```python
from build123d import *

# Parameters (mm, degrees)
SKETCH1_W                       = 314
SKETCH1_H                       = 134
BOSS_EXTRUDE1_DEPTH             = 160
SKETCH2_W                       = 350
SKETCH2_H                       = 150
BOSS_EXTRUDE3_DEPTH             = 10
SKETCH3_R                       = 41
BOSS_EXTRUDE5_DEPTH             = 150
F_5_0MM_DOWEL_HOLE1_D           = 5
F_5_0MM_DOWEL_HOLE1_CSINK_D     = 5.05
F_5_0MM_DOWEL_HOLE1_CSINK_ANGLE = 100
CIRPATTERN1_COUNT               = 6
SKETCH3_3_R                     = 27.5
CUT_EXTRUDE1_DEPTH              = 151
SKETCH6_R                       = 43
BOSS_EXTRUDE6_DEPTH             = 150
SKETCH6_3_R                     = 27.5
CUT_EXTRUDE2_DEPTH              = 151
F_5_0MM_DOWEL_HOLE2_D           = 5
F_5_0MM_DOWEL_HOLE2_CSINK_D     = 5.05
F_5_0MM_DOWEL_HOLE2_CSINK_ANGLE = 100
CIRPATTERN2_COUNT               = 6
MIRROR1_COPY_1_D                = 5
MIRROR1_COPY_1_CSINK_D          = 5.05
MIRROR1_COPY_1_CSINK_ANGLE      = 100
MIRROR1_COPY_2_D                = 5
MIRROR1_COPY_2_CSINK_D          = 5.05
MIRROR1_COPY_2_CSINK_ANGLE      = 100
MIRROR1_COPY_3_D                = 5
MIRROR1_COPY_3_CSINK_D          = 5.05
MIRROR1_COPY_3_CSINK_ANGLE      = 100
MIRROR1_COPY_4_D                = 5
MIRROR1_COPY_4_CSINK_D          = 5.05
MIRROR1_COPY_4_CSINK_ANGLE      = 100
MIRROR1_COPY_5_D                = 5
MIRROR1_COPY_5_CSINK_D          = 5.05
MIRROR1_COPY_5_CSINK_ANGLE      = 100
MIRROR2_COPY_1_D                = 5
MIRROR2_COPY_1_CSINK_D          = 5.05
MIRROR2_COPY_1_CSINK_ANGLE      = 100
MIRROR2_COPY_2_D                = 5
MIRROR2_COPY_2_CSINK_D          = 5.05
MIRROR2_COPY_2_CSINK_ANGLE      = 100
MIRROR2_COPY_3_D                = 5
MIRROR2_COPY_3_CSINK_D          = 5.05
MIRROR2_COPY_3_CSINK_ANGLE      = 100
MIRROR2_COPY_4_D                = 5
MIRROR2_COPY_4_CSINK_D          = 5.05
MIRROR2_COPY_4_CSINK_ANGLE      = 100
MIRROR2_COPY_5_D                = 5
MIRROR2_COPY_5_CSINK_D          = 5.05
MIRROR2_COPY_5_CSINK_ANGLE      = 100
SKETCH9_R                       = 12.5
BOSS_EXTRUDE7_DEPTH             = 6
CUT_EXTRUDE3_START              = 6
SKETCH9_3_R                     = 9
CUT_EXTRUDE3_DEPTH              = 30
CHAMFER1_SIZE                   = 2
SKETCH10_W                      = 26.35
SKETCH10_H                      = 43
BOSS_EXTRUDE8_DEPTH             = 25
CUT_EXTRUDE4_REACH              = 90.175
SKETCH12_R                      = 7.5
CUT_EXTRUDE5_DEPTH              = 50
CUT_EXTRUDE6_START              = -161
SKETCH13_R                      = 4
CUT_EXTRUDE6_DEPTH              = 205
MIRROR5_START                   = -161
MIRROR5_COPY_1_SKETCH_R         = 4
MIRROR5_COPY_1_DEPTH            = 205
MIRROR5_COPY_2_SKETCH_R         = 4
MIRROR5_COPY_2_DEPTH            = 205
SKETCH14_W                      = 364.166364604
SKETCH14_H                      = 92.820269588
CUT_EXTRUDE7_DEPTH              = 151
SKETCH15_W                      = 300
SKETCH15_H                      = 120
CUT_EXTRUDE9_DEPTH              = 150


with BuildPart() as part:
    # Sketch1 → Boss-Extrude1 (new body)
    with BuildSketch(Plane(origin=(0, 0, 0), x_dir=(1, 0, 0), z_dir=(0, 1, 0))):
        Rectangle(SKETCH1_W, SKETCH1_H)
    extrude(amount=BOSS_EXTRUDE1_DEPTH)

    # Sketch2 → Boss-Extrude3 (add)
    with BuildSketch(Plane(origin=(0, 160, 0), x_dir=(1, 0, 0), z_dir=(0, 1, 0))):
        Rectangle(SKETCH2_W, SKETCH2_H)
    extrude(amount=-BOSS_EXTRUDE3_DEPTH)

    # Sketch3 → Boss-Extrude5 (add, through all)
    with BuildSketch(Plane.XY.offset(75)):
        with Locations((95, 160)):
            Circle(SKETCH3_R)
    extrude(amount=-BOSS_EXTRUDE5_DEPTH)

    # Ø5.0mm Dowel Hole1 (through all)
    with Locations(Plane.XY.offset(75)):
        with Locations((95, 195)):
            f_5_0mm_dowel_hole1 = CounterSinkHole(F_5_0MM_DOWEL_HOLE1_D / 2, F_5_0MM_DOWEL_HOLE1_CSINK_D / 2, counter_sink_angle=F_5_0MM_DOWEL_HOLE1_CSINK_ANGLE)

    # CirPattern1: Ø5.0mm Dowel Hole1 ×6 about axis
    cirpattern1_axis = Axis((95, 160, 0), (0, 0, 1))
    for i in range(1, CIRPATTERN1_COUNT):
        add(f_5_0mm_dowel_hole1.rotate(cirpattern1_axis, i * 360 / CIRPATTERN1_COUNT), mode=Mode.SUBTRACT)

    # Sketch3<3> → Cut-Extrude1 (cut, through all)
    with BuildSketch(Plane.XY.offset(75)):
        with Locations((95, 160)):
            Circle(SKETCH3_3_R)
    extrude(amount=-CUT_EXTRUDE1_DEPTH, mode=Mode.SUBTRACT)

    # Sketch6 → Boss-Extrude6 (add, through all)
    with BuildSketch(Plane.XY.offset(75)):
        with Locations((-25, 160)):
            Circle(SKETCH6_R)
    extrude(amount=-BOSS_EXTRUDE6_DEPTH)

    # Sketch6<3> → Cut-Extrude2 (cut, through all)
    with BuildSketch(Plane.XY.offset(75)):
        with Locations((-25, 160)):
            Circle(SKETCH6_3_R)
    extrude(amount=-CUT_EXTRUDE2_DEPTH, mode=Mode.SUBTRACT)

    # Ø5.0mm Dowel Hole2 (through all)
    with Locations(Plane.XY.offset(75)):
        with Locations((-25, 193)):
            f_5_0mm_dowel_hole2 = CounterSinkHole(F_5_0MM_DOWEL_HOLE2_D / 2, F_5_0MM_DOWEL_HOLE2_CSINK_D / 2, counter_sink_angle=F_5_0MM_DOWEL_HOLE2_CSINK_ANGLE)

    # CirPattern2: Ø5.0mm Dowel Hole2 ×6 about axis
    cirpattern2_axis = Axis((-25, 160, 0), (0, 0, 1))
    for i in range(1, CIRPATTERN2_COUNT):
        add(f_5_0mm_dowel_hole2.rotate(cirpattern2_axis, i * 360 / CIRPATTERN2_COUNT), mode=Mode.SUBTRACT)

    # Mirror1: Ø5.0mm Dowel Hole2 across plane
    add(f_5_0mm_dowel_hole2.mirror(Plane.XY), mode=Mode.SUBTRACT)

    # Mirror1 copy 1 (through all)
    with Locations(Plane(origin=(126.064064606, 101.650635095, -75), x_dir=(0.5, 0.866025404, 0), z_dir=(0, 0, -1))):
        with Locations((-25, -193)):
            CounterSinkHole(MIRROR1_COPY_1_D / 2, MIRROR1_COPY_1_CSINK_D / 2, counter_sink_angle=MIRROR1_COPY_1_CSINK_ANGLE)

    # Mirror1 copy 2 (through all)
    with Locations(Plane(origin=(101.064064606, 261.650635095, -75), x_dir=(-0.5, 0.866025404, 0), z_dir=(0, 0, -1))):
        with Locations((-25, -193)):
            CounterSinkHole(MIRROR1_COPY_2_D / 2, MIRROR1_COPY_2_CSINK_D / 2, counter_sink_angle=MIRROR1_COPY_2_CSINK_ANGLE)

    # Mirror1 copy 3 (through all)
    with Locations(Plane(origin=(-50, 320, -75), x_dir=(-1, 0, 0), z_dir=(0, 0, -1))):
        with Locations((-25, -193)):
            CounterSinkHole(MIRROR1_COPY_3_D / 2, MIRROR1_COPY_3_CSINK_D / 2, counter_sink_angle=MIRROR1_COPY_3_CSINK_ANGLE)

    # Mirror1 copy 4 (through all)
    with Locations(Plane(origin=(-176.064064606, 218.349364905, -75), x_dir=(-0.5, -0.866025404, 0), z_dir=(0, 0, -1))):
        with Locations((-25, -193)):
            CounterSinkHole(MIRROR1_COPY_4_D / 2, MIRROR1_COPY_4_CSINK_D / 2, counter_sink_angle=MIRROR1_COPY_4_CSINK_ANGLE)

    # Mirror1 copy 5 (through all)
    with Locations(Plane(origin=(-151.064064606, 58.349364905, -75), x_dir=(0.5, -0.866025404, 0), z_dir=(0, 0, -1))):
        with Locations((-25, -193)):
            CounterSinkHole(MIRROR1_COPY_5_D / 2, MIRROR1_COPY_5_CSINK_D / 2, counter_sink_angle=MIRROR1_COPY_5_CSINK_ANGLE)

    # Mirror2: Ø5.0mm Dowel Hole1 across plane
    add(f_5_0mm_dowel_hole1.mirror(Plane.XY), mode=Mode.SUBTRACT)

    # Mirror2 copy 1 (through all)
    with Locations(Plane(origin=(186.064064606, -2.27241336, -75), x_dir=(0.5, 0.866025404, 0), z_dir=(0, 0, -1))):
        with Locations((95, -195)):
            CounterSinkHole(MIRROR2_COPY_1_D / 2, MIRROR2_COPY_1_CSINK_D / 2, counter_sink_angle=MIRROR2_COPY_1_CSINK_ANGLE)

    # Mirror2 copy 2 (through all)
    with Locations(Plane(origin=(281.064064606, 157.72758664, -75), x_dir=(-0.5, 0.866025404, 0), z_dir=(0, 0, -1))):
        with Locations((95, -195)):
            CounterSinkHole(MIRROR2_COPY_2_D / 2, MIRROR2_COPY_2_CSINK_D / 2, counter_sink_angle=MIRROR2_COPY_2_CSINK_ANGLE)

    # Mirror2 copy 3 (through all)
    with Locations(Plane(origin=(190, 320, -75), x_dir=(-1, 0, 0), z_dir=(0, 0, -1))):
        with Locations((95, -195)):
            CounterSinkHole(MIRROR2_COPY_3_D / 2, MIRROR2_COPY_3_CSINK_D / 2, counter_sink_angle=MIRROR2_COPY_3_CSINK_ANGLE)

    # Mirror2 copy 4 (through all)
    with Locations(Plane(origin=(3.935935394, 322.27241336, -75), x_dir=(-0.5, -0.866025404, 0), z_dir=(0, 0, -1))):
        with Locations((95, -195)):
            CounterSinkHole(MIRROR2_COPY_4_D / 2, MIRROR2_COPY_4_CSINK_D / 2, counter_sink_angle=MIRROR2_COPY_4_CSINK_ANGLE)

    # Mirror2 copy 5 (through all)
    with Locations(Plane(origin=(-91.064064606, 162.27241336, -75), x_dir=(0.5, -0.866025404, 0), z_dir=(0, 0, -1))):
        with Locations((95, -195)):
            CounterSinkHole(MIRROR2_COPY_5_D / 2, MIRROR2_COPY_5_CSINK_D / 2, counter_sink_angle=MIRROR2_COPY_5_CSINK_ANGLE)

    # Sketch9 → Boss-Extrude7 (add)
    with BuildSketch(Plane(origin=(157, 0, 0), x_dir=(0, 0, -1), z_dir=(1, 0, 0))):
        with Locations((0, 22.5)):
            Circle(SKETCH9_R)
    extrude(amount=BOSS_EXTRUDE7_DEPTH)

    # Sketch9<3> → Cut-Extrude3 (cut)
    with BuildSketch(Plane(origin=(157, 0, 0), x_dir=(0, 0, -1), z_dir=(1, 0, 0)).offset(CUT_EXTRUDE3_START)):
        with Locations((0, 22.5)):
            Circle(SKETCH9_3_R)
    extrude(amount=-CUT_EXTRUDE3_DEPTH, mode=Mode.SUBTRACT)

    # Chamfer1
    chamfer1_edges = [part.edges().sort_by_distance(p)[0] for p in [
        (163, 22.5, 12.5),
    ]]
    chamfer(chamfer1_edges, length=CHAMFER1_SIZE)

    # Sketch10 → Boss-Extrude8 (add)
    with BuildSketch(Plane(origin=(157, 0, 0), x_dir=(0, 0, -1), z_dir=(1, 0, 0))):
        with Locations((0, 66.5)):
            Rectangle(SKETCH10_W, SKETCH10_H)
    extrude(amount=BOSS_EXTRUDE8_DEPTH)

    # Sketch11 → Cut-Extrude4 (cut, up to next)
    with BuildSketch(Plane(origin=(0, 0, -13.175), x_dir=(-1, 0, 0), z_dir=(0, 0, -1)), mode=Mode.PRIVATE) as cut_extrude4_sk1:
        Polygon((-162, 88), (-182, 68), (-200.649139224, 72.819299993), (-183.741650688, 106.337654458), align=None)
    cut_extrude4_tool1 = extrude(cut_extrude4_sk1.sketch, amount=-CUT_EXTRUDE4_REACH, mode=Mode.PRIVATE) & part.part
    add(cut_extrude4_tool1.solids().sort_by_distance((181.949584, 85.075168, -13.175))[0], mode=Mode.SUBTRACT)

    # Sketch12 → Cut-Extrude5 (cut)
    with BuildSketch(Plane(origin=(125, 125, 0), x_dir=(0, 0, -1), z_dir=(0.707106781, 0.707106781, 0))):
        with Locations((0, -63.993163697)):
            Circle(SKETCH12_R)
    extrude(amount=-CUT_EXTRUDE5_DEPTH, mode=Mode.SUBTRACT)

    # Sketch13 → Cut-Extrude6 (cut)
    with BuildSketch(Plane(origin=(0, 160, 0), x_dir=(1, 0, 0), z_dir=(0, 1, 0)).offset(CUT_EXTRUDE6_START)):
        with Locations((-167, 67)):
            Circle(SKETCH13_R)
    cut_extrude6 = extrude(amount=CUT_EXTRUDE6_DEPTH, mode=Mode.SUBTRACT)

    # Mirror3: Cut-Extrude6 across plane
    add(cut_extrude6.mirror(Plane(origin=(0, 0, 0), x_dir=(0, 0, 1), z_dir=(1, 0, 0))), mode=Mode.SUBTRACT)

    # Mirror4: Cut-Extrude6 across plane
    add(cut_extrude6.mirror(Plane.XY), mode=Mode.SUBTRACT)

    # Mirror5 copy 1 sketch → Mirror5 copy 1 (cut)
    with BuildSketch(Plane(origin=(0, 160, 0), x_dir=(-1, 0, 0), z_dir=(0, 1, 0)).offset(MIRROR5_START)):
        with Locations((-167, 67)):
            Circle(MIRROR5_COPY_1_SKETCH_R)
    extrude(amount=MIRROR5_COPY_1_DEPTH, mode=Mode.SUBTRACT)

    # Mirror5 copy 2 sketch → Mirror5 copy 2 (cut)
    with BuildSketch(Plane(origin=(0, 160, 0), x_dir=(1, 0, 0), z_dir=(0, 1, 0)).offset(MIRROR5_START)):
        with Locations((-167, -67)):
            Circle(MIRROR5_COPY_2_SKETCH_R)
    extrude(amount=MIRROR5_COPY_2_DEPTH, mode=Mode.SUBTRACT)

    # Sketch14 → Cut-Extrude7 (cut, through all)
    with BuildSketch(Plane.XY.offset(75)):
        with Locations((7.083182302, 206.410134794)):
            Rectangle(SKETCH14_W, SKETCH14_H)
    extrude(amount=-CUT_EXTRUDE7_DEPTH, mode=Mode.SUBTRACT)

    # Sketch15 → Cut-Extrude9 (cut)
    with BuildSketch(Plane(origin=(0, 160, 0), x_dir=(1, 0, 0), z_dir=(0, 1, 0))):
        Rectangle(SKETCH15_W, SKETCH15_H)
    extrude(amount=-CUT_EXTRUDE9_DEPTH, mode=Mode.SUBTRACT)


solid = part.part
```
Part model, mm, in its own coordinate system. A direction names the side the tool comes from. Round coordinates to 2 decimals unless told otherwise and drop trailing zeros. Write each loop counter-clockwise with the first axis right and the second up, starting at its lowest first coordinate (ties: lowest second). Pieces come first, ordered by that corner, then holes. Notation, with made-up numbers: (-18.75, 78) -> (32.25, 78) arc R14 cw to (32.25, 89) -> close; hole circle Ø6 at (85.25, 9). An arc over 180 degrees is marked (long way). Return JSON: item names as keys, results as strings. Group by question number.
Q1. Probe L1, parallel to Y at x = 95, z = 69.5; L2, parallel to X at y = 136, z = 21.5; L3, parallel to Z at x = 12.5, y = 82.5. List the from-to ranges inside material, lowest first. Write a range as [from, to].
Q2. Saw through at D-D on z = 0. State how many separate pieces and enclosed holes the cut face has, plus the area to 3 significant figures.
Q3. Which spindle directions (+Z, -Z, +X, -X, +Y, -Y) get a long thin tool onto all of the face, cutting with end or side? Do faces 4 (the cylindrical face through (158.972, 10.297, 2.71)), 5 (the flat face through (35, 160, -68)), 6 (the cylindrical face through (94.24, 119.007, -70.944)), 7 (the flat face through (169, 45, 0)), 8 (the flat face through (-2, 86, 60)). Say none if no direction does.
Q4. Mould opens along Z. For faces 1 (the flat face through (12, 143, -75)), 2 (the cylindrical face through (-25.605, 132.507, 67.605)), 3 (the flat face through (-2, 10, -1)) say: pulls with the +Z half, pulls with the -Z half, needs draft (parallel to the pull), parting line crosses it, or undercut.
Q5. Saw through at C-C on x = -137.5. Write the cut outline in (y, z), plus the area to 3 significant figures.
Q6. Pin check, flat tips, straight feed: pin 1 (5 mm diameter, centred on x = 167, z = 67, fed in from -Y); pin 2 (11 mm diameter, centred on y = 22.5, z = 0, fed in from -X); pin 3 (6.5 mm diameter, centred on y = 26.5, z = 0, fed in from +X); pin 4 (4 mm diameter, centred on x = 28, z = 72, fed in from -Y). Stop position of each tip, or through.
Q7. Saw through at A-A on z = 55. Write the cut outline in (x, y), plus the area to 3 significant figures.
Q8. Saw through at B-B on y = 113. Write the cut outline in (x, z), plus the area to 3 significant figures.
Answer:
{
 "1": {"L1": "[119, 122.5], [127.5, 132.5]", "L2": "[-157, -150], [150, 157]", "L3": "[-67, -60], [60, 67]"},
 "2": {"separate pieces": "3", "enclosed holes": "0", "area": "5,960 mm2"},
 "3": {"face 4": "+X", "face 5": "+Z, -Z, +X, -X, +Y", "face 6": "-Z, -Y", "face 7": "+Z, -Z, +X", "face 8": "+Y"},
 "4": {"face 1": "pulls with the -Z half", "face 2": "needs draft", "face 3": "undercut"},
 "5": {"outline": "(0, -67) -> (150, -67) -> (150, -75) -> (160, -75) -> (160, -60) -> (10, -60) -> (10, 60) -> (160, 60) -> (160, 75) -> (150, 75) -> (150, 67) -> (0, 67) -> close", "area": "3,600 mm2"},
 "6": {"pin 1": "through", "pin 2": "x = -157", "pin 3": "x = -150", "pin 4": "y = 150"},
 "7": {"outline": "(-175, 150) -> (-157, 150) -> (-157, 0) -> (157, 0) -> (157, 150) -> (175, 150) -> (175, 160) -> (150, 160) -> (150, 10) -> (-150, 10) -> (-150, 160) -> (-175, 160) -> close", "area": "5,600 mm2"},
 "8": {"outline": "(-157, -67) -> (157, -67) -> (157, 67) -> (-157, 67) -> close; hole (-150, -60) -> (150, -60) -> (150, 60) -> (-150, 60) -> close", "area": "6,080 mm2"}
}
